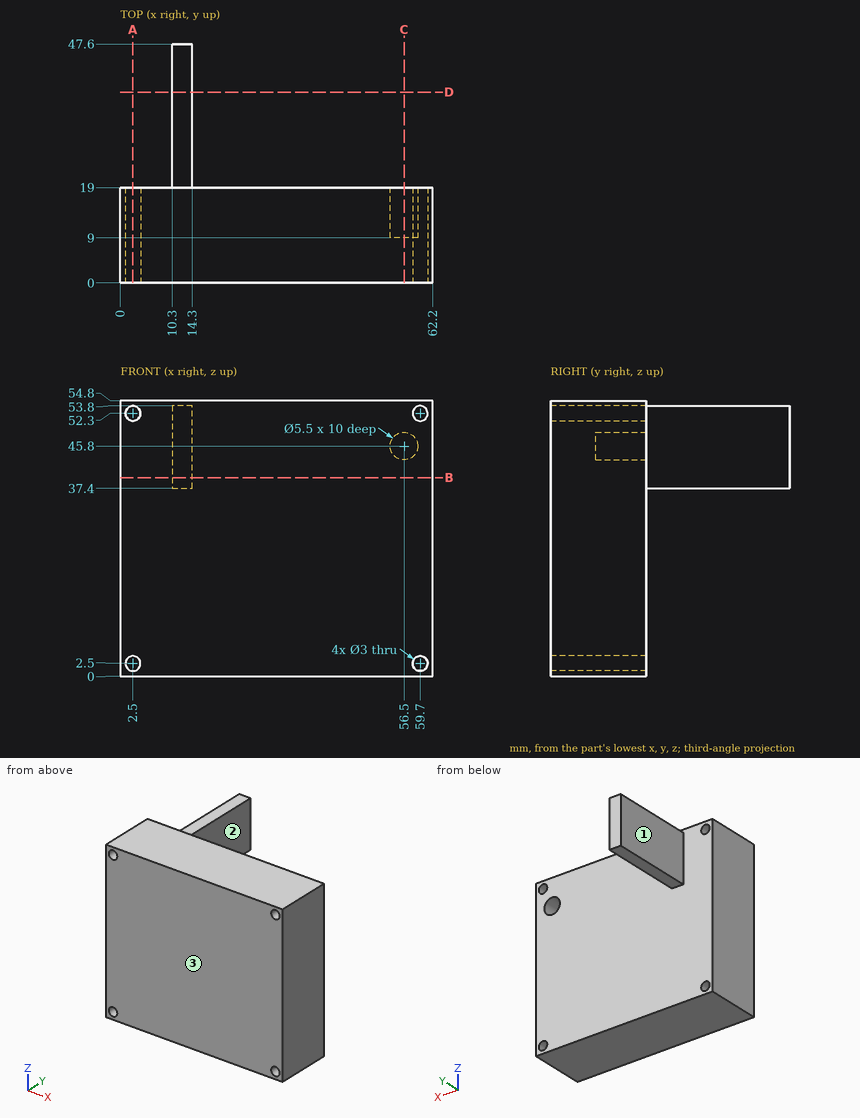
Geometry check sheet. Reference: drawing and pictorial views, mm from the part's lowest x, y, z. A direction names the side the tool comes from. Round coordinates to 2 decimals unless told otherwise and drop trailing zeros. Order: outer loops, then holes, each group sorted by start corner. A loop starts at its lowest first (then second) coordinate and runs counter-clockwise, first axis right, second up. Notation, with made-up numbers: M -5.5,-34 L 43.5,-34 A19 cw 43.5,2 Z; hole C 85,37 d6. An arc over 180 degrees is marked long. Write item = value, one per line.
Q1. Section check C-C (x = 56.5). Enter the section's corners in (y, z).
Answer block:
outline = M 0,0 L 19,0 L 19,43.05 L 9,43.05 L 9,48.55 L 19,48.55 L 19,54.8 L 0,54.8 Z
Q2. Section check A-A (x = 2.5). Enter the section's corners in (y, z).
Answer block:
outline = M 0,0 L 19,0 L 19,1 L 0,1 Z; M 0,4 L 19,4 L 19,50.8 L 0,50.8 Z; M 0,53.8 L 19,53.8 L 19,54.8 L 0,54.8 Z
Q3. Set-up check for the marked faces 1, 2 and 3: record each of +Z, -Z, +X, -X, +Y, -Y from which the full face is reachable in a straight line by a thin tool's end or side.
Answer block:
face_1 = +Z, -Z, -X, +Y
face_2 = +Z, -Z, +X, +Y
face_3 = +Z, -Z, +X, -X, -Y
Q4. Depth check by flat-ended pin: pin 1 Ø5 at (x, z) = (35, 47) entering from +Y; pin 2 Ø1 at (y, z) = (8, 11) entering from -X; pin 3 Ø3 at (x, y) = (12, 38) entering from +Z; pin 4 Ø2.5 at (x, z) = (2.5, 2.5) entering from -Y. Enter the tip coordinate at first touch or a pass-through.
Answer block:
pin_1 = 19
pin_2 = 0
pin_3 = 53.8
pin_4 = through
Q5. Section check B-B (z = 39.5). Enter the section's corners in (x, y), plus the area to 3 significant figures.
Answer block:
outline = M 0,0 L 62.2,0 L 62.2,19 L 14.3,19 L 14.3,47.6 L 10.3,47.6 L 10.3,19 L 0,19 Z
area = 1,300 mm^2
Q6. Section check D-D (y = 38). Enter the section's corners in (x, z), plus the area to 3 significant figures.
Answer block:
outline = M 10.3,37.4 L 14.3,37.4 L 14.3,53.8 L 10.3,53.8 Z
area = 65.6 mm^2
Q7. Scan lines: line 1 (X direction, y = 4.25, z = 2.5); line 2 (Z direction, x = 56.5, y = 11.5); line 3 (Z direction, x = 59, y = 4). Record each from-to range of solid material in increasing order.
Answer block:
line_1 = 0 to 1, 4 to 58.2, 61.2 to 62.2
line_2 = 0 to 43.05, 48.55 to 54.8
line_3 = 0 to 1.17, 3.83 to 50.97, 53.63 to 54.8
